```python
from build123d import *

# Parameters (mm, degrees)
SKETCH1_W           = 22
SKETCH1_H           = 166.3
SKETCH1_R           = 1.5
BOSS_EXTRUDE1_DEPTH = 5
CUT_EXTRUDE1_DEPTH  = 5


with BuildPart() as part:
    # Sketch1 → Boss-Extrude1 (new body)
    with BuildSketch(Plane(origin=(0, 0, 0), x_dir=(1, 0, 0), z_dir=(0, 1, 0))):
        with Locations((11, 83.15)):
            Rectangle(SKETCH1_W, SKETCH1_H)
        with Locations(Location((5, 161.3, 0), (0, 0, 270))):
            Circle(SKETCH1_R, mode=Mode.SUBTRACT)
        with Locations(Location((17, 161.3, 0), (0, 0, 270))):
            Circle(SKETCH1_R, mode=Mode.SUBTRACT)
        with Locations(Location((17, 5, 0), (0, 0, 270))):
            Circle(SKETCH1_R, mode=Mode.SUBTRACT)
        with Locations(Location((5, 5, 0), (0, 0, 270))):
            Circle(SKETCH1_R, mode=Mode.SUBTRACT)
    extrude(amount=BOSS_EXTRUDE1_DEPTH)

    # Sketch2 → Cut-Extrude1 (cut)
    with BuildSketch(Plane(origin=(0, 0, 0), x_dir=(-1, 0, 0), z_dir=(0, -1, 0))):
        with BuildLine():
            Line((-16, 40), (-16, 60))
            ThreePointArc((-16, 60), (-11, 65), (-6, 60))
            Line((-6, 60), (-6, 40))
            ThreePointArc((-6, 40), (-11, 35), (-16, 40))
        make_face()
    extrude(amount=-CUT_EXTRUDE1_DEPTH, mode=Mode.SUBTRACT)


solid = part.part
```
Check sheet for the modelled part. Datum: model origin and axes. Units: mm. A direction names the side the tool comes from. Coordinates: 2 decimals unless noted, no trailing zeros. Loops run counter-clockwise (first coordinate to the right, second up) from the corner with the lowest first, then second, coordinate; pieces in that order, holes last.
1) Sectioned sample at D-D (z = -161.3). Record the boundary of the cut face in (x, y).
2) Sectioned sample at C-C (x = 8.75). Record the boundary of the cut face in (y, z).
3) Access from +Z, -Z, +X, -X, +Y, -Y to the whole of each face (thin tool, end or side, straight path). Record for faces 1 (the face through (11, 0, -84)), 2 (the face through (11, 2, -35)).
4) Release check for a two-part mould opening along Z. For faces 3 (the face through (11, 5, -84)), 4 (the face through (6, 2, -50)), 5 (the face through (11, 2, -166.3)) record: released by +Z, released by -Z, zero draft, split by the parting line, or undercut.
5) Sectioned sample at A-A (y = 1.7). Record the boundary of the cut face in (x, z), and give its area (3 significant figures).
6) Sectioned sample at B-B (z = -63). Record the boundary of the cut face in (x, y), and give its area (3 significant figures).
7) Material ranges on probe 1 along X at (y, z) = (1.65, -161.3); probe 2 along Z at (x, y) = (11.25, 1.4); probe 3 along Z at (x, y) = (16.5, 3.2), recorded low to high.
Check sheet entries:
1. outline: (0, 0) - (3.5, 0) - (3.5, 5) - (0, 5) - close; (6.5, 0) - (15.5, 0) - (15.5, 5) - (6.5, 5) - close; (18.5, 0) - (22, 0) - (22, 5) - (18.5, 5) - close
2. outline: (0, -166.3) - (5, -166.3) - (5, -64.47) - (0, -64.47) - close; (0, -35.53) - (5, -35.53) - (5, 0) - (0, 0) - close
3. face 1: +Z, -Z, +X, -X, -Y
3. face 2: +Y, -Y
4. face 3: zero draft
4. face 4: undercut
4. face 5: released by -Z
5. outline: (0, -166.3) - (22, -166.3) - (22, 0) - (0, 0) - close; hole circle Ø3 at (5, -161.3); hole circle Ø3 at (5, -5); hole (6, -60) arc R5 ccw to (16, -60) - (16, -40) arc R5 ccw to (6, -40) - close; hole circle Ø3 at (17, -161.3); hole circle Ø3 at (17, -5)
5. area: 3,350 mm2
6. outline: (0, 0) - (7, 0) - (7, 5) - (0, 5) - close; (15, 0) - (22, 0) - (22, 5) - (15, 5) - close
6. area: 70.0 mm2
7. probe 1: x = 0 to 3.5, 6.5 to 15.5, 18.5 to 22
7. probe 2: z = -166.3 to -64.99, -35.01 to 0
7. probe 3: z = -166.3 to -162.71, -159.89 to -6.41, -3.59 to 0
